from build123d import *

# Parameters (mm, degrees)
SKETCH1_R           = 3.175
BOSS_EXTRUDE1_DEPTH = 5.842
FILLET1_R           = 25.4
SKETCH2_W           = 6.35
SKETCH2_H           = 6.35
BOSS_EXTRUDE2_DEPTH = 5.842
FILLET4_R           = 1.5875
FILLET5_R           = 25.4
FILLET6_R           = 6.35
SKETCH3_W           = 12.7
SKETCH3_H           = 5.842
CUT_EXTRUDE1_DEPTH  = 162.480283814
BOSS_EXTRUDE3_DEPTH = 5.842
FILLET7_R           = 6.35
FILLET8_R           = 1.5875
CUT_EXTRUDE2_DEPTH  = 162.480283814
BOSS_EXTRUDE4_DEPTH = 5.842
FILLET9_R           = 6.35
FILLET10_R          = 50.8


with BuildPart() as part:
    # Sketch1 → Boss-Extrude1 (new body)
    with BuildSketch(Plane.XY):
        with BuildLine():
            Line((44.45, -9.525), (-44.45, -9.525))
            ThreePointArc((-44.45, -9.525), (-51.185192091, -6.735192091), (-53.975, 0))
            Line((-53.975, 0), (-158.75, 19.05))
            Line((-158.75, 19.05), (-158.75, 22.225))
            Line((-158.75, 22.225), (44.45, 20.921420052))
            Line((44.45, 20.921420052), (44.45, 9.525))
            ThreePointArc((44.45, 9.525), (53.975, 0), (44.45, -9.525))
        make_face()
        with Locations((44.45, 0)):
            Circle(SKETCH1_R, mode=Mode.SUBTRACT)
        with BuildLine():
            Line((19.05, -3.175), (-44.45, -3.175))
            ThreePointArc((-44.45, -3.175), (-47.625, 0), (-44.45, 3.175))
            Line((-44.45, 3.175), (19.05, 3.175))
            ThreePointArc((19.05, 3.175), (22.225, 0), (19.05, -3.175))
        make_face(mode=Mode.SUBTRACT)
    extrude(amount=BOSS_EXTRUDE1_DEPTH)

    # Fillet1
    # the kernel refuses this fillet: 25.4 mm, written as the material it adds along each edge
    with BuildSketch(Plane(origin=(44.45, 9.525, 0), x_dir=(0, 1, 0), z_dir=(0, 0, 1))) as fillet1_piece_1:
        with BuildLine():
            CenterArc((14.667942914, -25.188432626), FILLET1_R, 97.400260925, 36.444857628)
            Line((-2.92692466, -6.869572534), (-3.278822011, -6.503195333))
            ThreePointArc((-3.278822011, -6.503195333), (-1.229577289, -3.534437867), (-0.508, 0))
            Line((-0.508, 0), (0, 0.508))
            ThreePointArc((0, 0.508), (5.698210026, 0.508), (11.330989595, 0.503768653))
            Line((11.330989595, 0.503768653), (11.396420052, 0))
        make_face()
    extrude(amount=5.842)

    # Sketch2 → Boss-Extrude2 (add)
    with BuildSketch(Plane.XY.offset(5.842)):
        with Locations((-155.65673172, 25.359787457)):
            Rectangle(SKETCH2_W, SKETCH2_H)
    extrude(amount=-BOSS_EXTRUDE2_DEPTH)

    # Fillet4
    # the kernel refuses this fillet: 1.5875 mm, written as the material it adds along each edge
    with BuildSketch(Plane(origin=(-152.48173172, 22.184787457, 5.842), x_dir=(0.9999794228826333, -0.00641512363991872, 0), z_dir=(0, 0, -1))) as fillet4_piece_1:
        with BuildLine():
            CenterArc((FILLET4_R * 0.993605321893, -FILLET4_R), FILLET4_R, 90, 89.632437969)
            Line((-FILLET4_R * 0.00637410098923, -FILLET4_R * 0.99358487636), (0, 0))
            Line((0, 0), (FILLET4_R * 0.993605321893, 0))
        make_face()
    extrude(amount=5.842)
    # the kernel refuses this fillet: 1.5875 mm, written as the material it takes off along each edge
    with BuildSketch(Plane(origin=(-158.83173172, 28.534787457, 9.81075), x_dir=(0, -1, 0), z_dir=(0, 0, -1)), Plane(origin=(-152.48173172, 28.534787457, 9.81075), x_dir=(-1, 0, 0), z_dir=(0, 0, -1))) as fillet4_2_piece_1:
        with BuildLine():
            CenterArc((FILLET4_R, -FILLET4_R), FILLET4_R, 90, 90)
            Line((0, -FILLET4_R), (0, 0))
            Line((0, 0), (FILLET4_R, 0))
        make_face()
    extrude(amount=13.7795, mode=Mode.SUBTRACT)
    with BuildSketch(Plane(origin=(-158.83173172, 22.184787457, 7.099025602), x_dir=(1.0, 1.4344436985779291e-12, 0), z_dir=(0, 0, -1))) as fillet4_2_piece_2:
        with BuildLine():
            CenterArc((1.5875, -0.502810241), FILLET4_R, 161.534664076, 18.465335924)
            Line((0, -0.502810241), (0, 0))
            Line((0, 0), (0.08173172, 0))
        make_face()
    extrude(amount=8.356051205, mode=Mode.SUBTRACT)

    # Fillet5
    fillet5_edges = [part.edges().sort_by_distance(p)[0] for p in [
        (-53.975, 0, 2.921),
    ]]
    fillet(fillet5_edges, radius=FILLET5_R)

    # Fillet6
    # the kernel refuses this fillet: 6.35 mm, written as the material it takes off along each edge
    with BuildSketch(Plane(origin=(-158.75, 19.05, -12.212686772), x_dir=(0.9838699100999072, -0.17888543819998437, 0), z_dir=(0, 0, 1))) as fillet6_piece_1:
        with BuildLine():
            CenterArc((4.885074709, 6.35), FILLET6_R, 210.950382336, 59.049617664)
            Line((-0.560767828, 3.084223053), (0, 0))
            Line((0, 0), (4.885074709, 0))
        make_face()
    extrude(amount=30.267373544, mode=Mode.SUBTRACT)

    # Sketch3 → Cut-Extrude1 (cut, through all)
    with BuildSketch(Plane.XY.offset(5.842)):
        with Locations((-88.98173172, 18.897155596)):
            Rectangle(SKETCH3_W, SKETCH3_H)
        with Locations((-63.58173172, 18.897155596)):
            Rectangle(SKETCH3_W, SKETCH3_H)
    extrude(amount=-CUT_EXTRUDE1_DEPTH, mode=Mode.SUBTRACT)

    # Sketch4 → Boss-Extrude3 (add)
    with BuildSketch(Plane.XY.offset(5.842)):
        Polygon((44.45, 20.921420052), (48.170691966, 27.271420052), (54.520691966, 27.271420052), (46.540749413, 13.626153894), (43.362669871, 15.484739273), align=None)
    extrude(amount=-BOSS_EXTRUDE3_DEPTH)

    # Fillet7
    fillet7_edges = [part.edges().sort_by_distance(p)[0] for p in [
        (44.45, 20.921420052, 2.921),
        (46.540749413, 13.626153894, 2.921),
    ]]
    fillet(fillet7_edges, radius=FILLET7_R)

    # Fillet8
    fillet8_edges = [part.edges().sort_by_distance(p)[0] for p in [
        (48.170691966, 27.271420052, 2.921),
        (54.520691966, 27.271420052, 2.921),
    ]]
    fillet(fillet8_edges, radius=FILLET8_R)

    # Sketch5 → Cut-Extrude2 (cut, through all)
    with BuildSketch(Plane.XY.offset(5.842)):
        with BuildLine():
            Line((41.13300152, 12.211269778), (-9.665953162, 12.537158059))
            ThreePointArc((-9.665953162, 12.537158059), (-12.03187815, 14.933635073), (-9.635401136, 17.29956006))
            Line((-9.635401136, 17.29956006), (41.163553547, 16.97367178))
            ThreePointArc((41.163553547, 16.97367178), (43.529478534, 14.577194766), (41.13300152, 12.211269778))
        make_face()
    extrude(amount=-CUT_EXTRUDE2_DEPTH, mode=Mode.SUBTRACT)

    # Sketch6 → Boss-Extrude4 (add)
    with BuildSketch(Plane.XY.offset(5.842)):
        Polygon((-158.811165573, 22.432892862), (-157.831118293, 16.403681612), (-110.184513465, 10.219911539), align=None)
    extrude(amount=-BOSS_EXTRUDE4_DEPTH)

    # Fillet9
    fillet9_edges = [part.edges().sort_by_distance(p)[0] for p in [
        (-157.831118293, 16.403681612, 2.921),
    ]]
    fillet(fillet9_edges, radius=FILLET9_R)

    # Fillet10
    # the kernel refuses this fillet: 50.8 mm, written as the material it adds along each edge
    with BuildSketch(Plane(origin=(-110.184513465, 10.219911539, 5.842), x_dir=(-0.9916829703779194, 0.1287046474002651, 0), z_dir=(0, 0, -1))) as fillet10_piece_1:
        with BuildLine():
            CenterArc((FILLET10_R * 0.0254008846311, -FILLET10_R), FILLET10_R, 90, 2.910101208)
            Line((-FILLET10_R * 0.0253681282132, -FILLET10_R * 0.0012895778381), (0, 0))
            Line((0, 0), (FILLET10_R * 0.0254008846311, 0))
        make_face()
    extrude(amount=5.842)


solid = part.part
Verification items for the finished model (mm, model axes). A direction names the side the tool comes from. Give positions to 0.01 mm unless a question says otherwise; leave off trailing zeros. Write each loop counter-clockwise with the first axis right and the second up, starting at its lowest first coordinate (ties: lowest second). Pieces come first, ordered by that corner, then holes. Notation, with made-up numbers: M -26,65.5 L 23,65.5 A27 ccw 23,81.5 Z; hole C -27,73.5 d2. An arc over 180 degrees is marked long. Put each result on its own line as item: value. Start each with the question number.
1. Scan lines: line 1 along X through (y, z) = (18, 1.15); line 2 along X through (y, z) = (25.5, 1.6); line 3 along X through (y, z) = (16.5, 1.4). Record each from-to range of solid material in increasing order. Write a range as [from, to].
2. Section check D-D (x = 17). Record the cut outline in (y, z) (3 decimals), and give its area (3 significant figures).
3. Draft check along X on faces 4 (the face through (43.53, 14.63, 2.96)), 5 (the face through (50.777, 20.871, 2.962)), 6 (the face through (-12, -3.175, 3)), 7 (the face through (-38, 7, 0)). Enter one of: +X half, -X half, draft (parallel to the pull), parting line (faces both ways), or undercut.
4. Set-up check for faces 1 (the face through (-13, 3.175, 3)), 2 (the face through (-82.632, 19, 3)), 3 (the face through (1, -9.525, 3)): record each of +Z, -Z, +X, -X, +Y, -Y from which the full face is reachable in a straight line by a thin tool's end or side.
5. Section check C-C (z = 1.9). Give the number of separate pieces and of enclosed holes in the cut face, and give its area (3 significant figures).
6. Section check A-A (y = 0). Record the cut outline in (x, z) (3 decimals).
7. Go/stop test with flat-tipped pins: pin 1 Ø3 at (x, z) = (-47, 2) entering from -Y; pin 2 Ø2 at (x, z) = (50.5, 2) entering from +Y; pin 3 Ø1.8 at (x, z) = (-86.5, 2) entering from +Y. Record where each tip stops, or that it passes through.
8. Section check B-B (x = -29). Record the cut outline in (y, z) (3 decimals).
Answer list:
1. line 1: [-157.18, -95.33], [-82.63, -69.93], [-57.23, 49.1]
1. line 2: [-158.83, -152.48], [47.13, 53.33]
1. line 3: [-155.33, -95.33], [-82.63, -69.93], [-57.23, -11.43], [42.57, 48.23]
2. outline: M -9.525,0 L -3.175,0 L -3.175,5.842 L -9.525,5.842 Z; M 3.175,0 L 12.366,0 L 12.366,5.842 L 3.175,5.842 Z; M 17.129,0 L 21.098,0 L 21.098,5.842 L 17.129,5.842 Z
2. area: 114 mm2
3. face 4: undercut
3. face 5: +X half
3. face 6: undercut
3. face 7: draft
4. face 1: +Z, -Z
4. face 2: +Z, -Z, +Y
4. face 3: +Z, -Z, +X, -X, -Y
5. separate pieces: 1
5. enclosed holes: 3
5. area: 3,770 mm2
6. outline: M -59.626,0 L -47.625,0 L -47.625,5.842 L -59.626,5.842 Z; M 22.225,0 L 41.275,0 L 41.275,5.842 L 22.225,5.842 Z; M 47.625,0 L 53.975,0 L 53.975,5.842 L 47.625,5.842 Z
7. pin 1: y = -9.47
7. pin 2: y = 27.27
7. pin 3: y = 15.98
8. outline: M -9.525,0 L -3.175,0 L -3.175,5.842 L -9.525,5.842 Z; M 3.175,0 L 21.393,0 L 21.393,5.842 L 3.175,5.842 Z
